from build123d import *

# Parameters (mm, degrees)
EXTRUDE_4_DEPTH = 15


with BuildPart() as part:
    # ｽｹｯﾁ2 → ﾎﾞｽ - 押し出し4 (new body)
    with BuildSketch(Plane(origin=(0, 0, 0), x_dir=(1, 0, 0), z_dir=(0, 1, 0))):
        with BuildLine():
            ThreePointArc((-53.82643789, -36.437818048), (-56.846261527, -34.367935813), (-60.466933112, -34.910600109))
            Line((-60.466933112, -34.910600109), (-64.807406984, -37.416573868))
            ThreePointArc((-64.807406984, -37.416573868), (-67.177509772, -40.614402853), (-66.461234116, -44.529814279))
            ThreePointArc((-66.461234116, -44.529814279), (49.665387485, -62.716419588), (58.57572973, 54.487465409))
            Line((58.57572973, 54.487465409), (57.289371136, 55.838409315))
            Line((57.289371136, 55.838409315), (25.911523347, 88.791671712))
            ThreePointArc((25.911523347, 88.791671712), (19.306695871, 93.382511176), (11.427401304, 95))
            Line((11.427401304, 95), (0, 95))
            ThreePointArc((0, 95), (-15, 80), (0, 65))
            ThreePointArc((0, 65), (57.41714976, -30.467538684), (-53.82643789, -36.437818048))
        make_face()
    extrude(amount=EXTRUDE_4_DEPTH)


solid = part.part
Here's how the part is built. I have some questions about the finished solid (model axes, mm). Round coordinates to 2 decimals unless told otherwise and drop trailing zeros. Order: outer loops, then holes, each group sorted by start corner. A loop starts at its lowest first (then second) coordinate and runs counter-clockwise, first axis right, second up. Notation, with made-up numbers: M -38,38.5 L -26,38.5 A24 ccw -26,66.5 Z; hole C 53,41 d11. An arc over 180 degrees is marked long. Return JSON: item names as keys, results as strings. Group by question number.
1. If we section it at B-B on y = 4.25: List the corners of the cut face in (x, z) for me.
2. If we mould it in two halves opening along Z, with no side actions, what happens to faces 1 (the face through (58.27, 7.4, 28.8)), 2 (the face through (-67.164, 7.395, 40.559)), 3 (the face through (6, 7, -95))? For each: pulls with the +Z half, pulls with the -Z half, needs draft (parallel to the pull), parting line crosses it, or undercut.
3. If we section it at C-C on z = 41: List the corners of the cut face in (x, y) for me.
4. If we section it at A-A on x = 14.5: List the corners of the cut face in (y, z) for me, then the cut area to 3 significant figures.
5. Please list where these lines run through material, in increasing order: probe 1 along Z at (x, y) = (0, 4); probe 2 along X at (y, z) = (10.5, 0); probe 3 along Z at (x, y) = (-13, 6.75).
6. I'm going to push flat-ended pins straight in: pin 1 Ø8 at (x, y) = (-37, 5.5) entering from +Z; pin 2 Ø6 at (x, y) = (58, 5.5) entering from +Z; pin 3 Ø1 at (x, y) = (19.5, 12) entering from +Z. Where does each tip first touch, or does it pass through?
7. If we section it at D-D on z = 15: List the corners of the cut face in (x, y) for me, then the cut area to 3 significant figures.
Reply:
{
 "1": {"outline": "M -66.46,44.53 A5 ccw -64.81,37.42 L -60.47,34.91 A5 ccw -53.83,36.44 A65 cw long 0,-65 A15 ccw 0,-95 L 11.43,-95 A20 ccw 25.91,-88.79 L 58.58,-54.49 A80 ccw long Z"},
 "2": {"face 1": "undercut", "face 2": "parting line crosses it", "face 3": "pulls with the -Z half"},
 "3": {"outline": "M -67.25,0 L -50.44,0 L -50.44,15 L -67.25,15 Z; M 50.44,0 L 68.69,0 L 68.69,15 L 50.44,15 Z"},
 "4": {"outline": "M 0,-94.76 L 15,-94.76 L 15,-63.36 L 0,-63.36 Z; M 0,63.36 L 15,63.36 L 15,78.67 L 0,78.67 Z", "area": "701 mm^2"},
 "5": {"probe 1": "-95 to -65, 65 to 80", "probe 2": "65 to 80", "probe 3": "-87.48 to -72.52, 63.69 to 78.94"},
 "6": {"pin 1": "z = 72.88", "pin 2": "z = 58.09", "pin 3": "z = 77.71"},
 "7": {"outline": "M 63.25,0 L 78.58,0 L 78.58,15 L 63.25,15 Z", "area": "230 mm^2"}
}
